Design review of the part shown in the three views and the two pictorial views. Dimensions are in mm from the part's minimum x, y and z. A direction names the side the tool comes from. Give positions to 0.01 mm unless a question says otherwise; leave off trailing zeros. Order: outer loops, then holes, each group sorted by start corner. A loop starts at its lowest first (then second) coordinate and runs counter-clockwise, first axis right, second up. Notation, with made-up numbers: M -19,-37 L -1,-37 A30 ccw -1,2 Z; hole C 40.5,17 d8. An arc over 180 degrees is marked long. Answer as a JSON object with one key per item and string values.
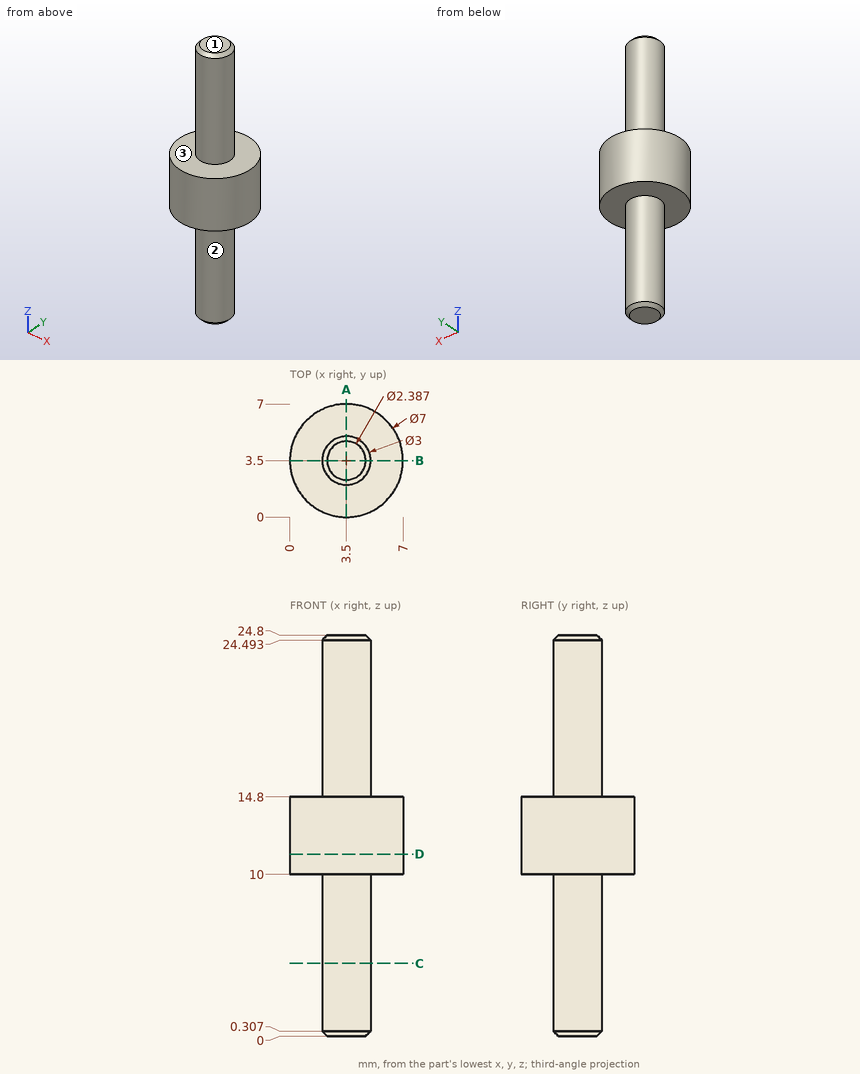
(1) We need section D-D (z = 11.25). Write out the cut boundary in (x, y), plus the area to 3 significant figures.
Checked values:
{"outline": "C 3.5,3.5 d7", "area": "38.5 mm^2"}
(2) We need section A-A (x = 3.5). Write out the cut boundary in (y, z).
Checked values:
{"outline": "M 0,10 L 2,10 L 2,0.31 L 2.31,0 L 4.69,0 L 5,0.31 L 5,10 L 7,10 L 7,14.8 L 5,14.8 L 5,24.49 L 4.69,24.8 L 2.31,24.8 L 2,24.49 L 2,14.8 L 0,14.8 Z"}
(3) To check wall thickness, follow L1, parallel to Z at x = 5, y = 0.5; L2, parallel to Y at x = 3.5, z = 23; L3, parallel to X at y = 1.25, z = 13. State the ranges of each line that lie inside material, in increasing order. Write a range as from..to.
Checked values:
{"L1": "z = 10..14.8", "L2": "y = 2..5", "L3": "x = 0.82..6.18"}
(4) Tool access review of the marked faces 1, 2 and 3: name each direction out of +Z, -Z, +X, -X, +Y, -Y from which nothing blocks a thin tool from reaching the whole face with its end or side.
Checked values:
{"face 1": "+Z, +X, -X, +Y, -Y", "face 2": "-Z", "face 3": "+Z"}
(5) Insertion check: pin 1 (1.5 mm diameter, centred on x = 6, y = 5.5, fed in from -Z); pin 2 (1 mm diameter, centred on x = 4.5, y = 6, fed in from +Z). Each pin has a flat end and moves straight along its axis. Give the tip position at first contact, or say it passes through.
Checked values:
{"pin 1": "stops at z = 10", "pin 2": "stops at z = 14.8"}
(6) We need section C-C (z = 4.5). Write out the cut boundary in (x, y).
Checked values:
{"outline": "C 3.5,3.5 d3"}
